Can you work these out from the model? Positions are in its coordinate system, mm. Give positions to 0.01 mm unless a question says otherwise; leave off trailing zeros. Order: outer loops, then holes, each group sorted by start corner. A loop starts at its lowest first (then second) coordinate and runs counter-clockwise, first axis right, second up. Notation, with made-up numbers: (48.25, 1.25) -> (94.25, 1.25) arc R36 ccw to (94.25, 37.25) -> close; hole circle Ø10 at (66, 10.25). An arc over 180 degrees is marked (long way). Answer as CSV lines item,"result".
```python
from build123d import *

# Parameters (mm, degrees)
BOSS_EXTRUDE1_DEPTH = 0.1
SKETCH2_R           = 0.1
BOSS_EXTRUDE2_DEPTH = 2
SKETCH3_R           = 2
BOSS_EXTRUDE3_DEPTH = 0.5


with BuildPart() as part:
    # Sketch1 → Boss-Extrude1 (new body)
    with BuildSketch(Plane(origin=(0, 0, 0), x_dir=(1, 0, 0), z_dir=(0, 1, 0))):
        with BuildLine():
            Line((-0.175, 0.46837485), (-0.175, 13))
            Line((-0.175, 13), (0.175, 13))
            Line((0.175, 13), (0.175, 0.46837485))
            Line((0.175, 0.46837485), (0.175, -0.46837485))
            Line((0.175, -0.46837485), (0.175, -2.53162515))
            ThreePointArc((0.175, -2.53162515), (0, -3.5), (-0.175, -2.53162515))
            Line((-0.175, -2.53162515), (-0.175, -0.46837485))
            Line((-0.175, -0.46837485), (-0.175, 0.46837485))
        make_face()
    extrude(amount=BOSS_EXTRUDE1_DEPTH)

    # Sketch2 → Boss-Extrude2 (add)
    with BuildSketch(Plane.XZ):
        Circle(SKETCH2_R)
    extrude(amount=BOSS_EXTRUDE2_DEPTH)

    # Sketch3 → Boss-Extrude3 (add)
    with BuildSketch(Plane.XZ.offset(2)):
        Circle(SKETCH3_R)
    extrude(amount=BOSS_EXTRUDE3_DEPTH)


solid = part.part
```
Item 1: Imagine slicing it at C-C, the plane y = -0.4. Please give me the cut outline in (x, z), then the cut area to 3 significant figures.
Numbers:
outline,"circle Ø0.2 at (0, 0)"
area,"0.0314 mm²"
Item 2: For pin 1 (1 mm diameter, centred on x = 1.5, y = -1, fed in from +Z); pin 2 (1.2 mm diameter, centred on x = 0.5, z = 0, fed in from +Y); pin 3 (2 mm diameter, centred on x = -1.5, z = 1, fed in from +Y), each with a flat end and sliding along its axis, tell me the tip position at first contact or that it passes through.
Numbers:
pin 1,"passes through"
pin 2,"stops at y = 0.1"
pin 3,"stops at y = -2"
Item 3: Please list where these lines run through material, in increasing order: line 1 along Y through (x, z) = (1.35, -0.5); line 2 along Z through (x, y) = (-1.4, -2.35).
Numbers:
line 1,"y = -2.5 to -2"
line 2,"z = -1.43 to 1.43"
Item 4: Imagine slicing it at B-B, the plane x = 0.8. Please give me the cut outline in (y, z).
Numbers:
outline,"(-2.5, -1.83) -> (-2, -1.83) -> (-2, 1.83) -> (-2.5, 1.83) -> close"
Item 5: Imagine slicing it at A-A, the plane z = -8. Please give me the cut outline in (x, y) (3 decimals), then the cut area to 3 significant figures.
Numbers:
outline,"(-0.175, 0) -> (0.175, 0) -> (0.175, 0.1) -> (-0.175, 0.1) -> close"
area,"0.0350 mm²"
